from build123d import *

# Parameters (mm, degrees)
SKETCH1_R           = 1.75
SKETCH1_R_2         = 1.798521792
BOSS_EXTRUDE1_DEPTH = 5
SKETCH2_R           = 2.65
CUT_EXTRUDE1_DEPTH  = 3.5


with BuildPart() as part:
    # Sketch1 → Boss-Extrude1 (new body)
    with BuildSketch(Plane.YZ):
        Polygon((-67.5, -15.65), (-67.5, 15.65), (-60.8, 22.35), (-29.12737367, 22.35), (-21.9, 29.57737367), (-21.9, 35.8), (-15.2, 42.5), (15.2, 42.5), (21.9, 35.8), (21.9, 29.57737367), (29.12737367, 22.35), (60.8, 22.35), (67.5, 15.65), (67.5, -15.65), (60.8, -22.35), (29.12737367, -22.35), (21.9, -29.57737367), (21.9, -35.8), (15.2, -42.5), (-15.2, -42.5), (-21.9, -35.8), (-21.9, -29.57737367), (-29.12737367, -22.35), (-60.8, -22.35), align=None)
        with Locations(Location((0, 32.15, 0), (0, 0, 270))):
            Circle(SKETCH1_R, mode=Mode.SUBTRACT)
        with Locations(Location((-32.15, 0, 0), (0, 0, 270))):
            Circle(SKETCH1_R, mode=Mode.SUBTRACT)
        with Locations(Location((0, -32.15, 0), (0, 0, 270))):
            Circle(SKETCH1_R, mode=Mode.SUBTRACT)
        with Locations(Location((32.15, 0, 0), (0, 0, 270))):
            Circle(SKETCH1_R, mode=Mode.SUBTRACT)
        with Locations(Location((-62.5, -15, 0), (0, 0, 270))):
            Circle(SKETCH1_R, mode=Mode.SUBTRACT)
        with Locations(Location((-62.5, 15, 0), (0, 0, 270))):
            Circle(SKETCH1_R, mode=Mode.SUBTRACT)
        with Locations(Location((62.5, -15, 0), (0, 0, 90))):
            Circle(SKETCH1_R, mode=Mode.SUBTRACT)
        with Locations(Location((62.5, 15, 0), (0, 0, 90))):
            Circle(SKETCH1_R, mode=Mode.SUBTRACT)
        with Locations(Location((-15, 30, 0), (0, 0, 270))):
            Circle(SKETCH1_R_2, mode=Mode.SUBTRACT)
        with Locations(Location((15, 30, 0), (0, 0, 270))):
            Circle(SKETCH1_R_2, mode=Mode.SUBTRACT)
        with Locations(Location((15, -30, 0), (0, 0, 270))):
            Circle(SKETCH1_R_2, mode=Mode.SUBTRACT)
        with Locations(Location((-15, -30, 0), (0, 0, 270))):
            Circle(SKETCH1_R_2, mode=Mode.SUBTRACT)
        with BuildLine():
            Line((41, -16), (47.5, -16))
            ThreePointArc((47.5, -16), (49.621320344, -15.121320344), (50.5, -13))
            Line((50.5, -13), (50.5, 13))
            ThreePointArc((50.5, 13), (49.621320344, 15.121320344), (47.5, 16))
            Line((47.5, 16), (41, 16))
            ThreePointArc((41, 16), (38.878679656, 15.121320344), (38, 13))
            Line((38, 13), (38, -13))
            ThreePointArc((38, -13), (38.878679656, -15.121320344), (41, -16))
        make_face(mode=Mode.SUBTRACT)
        with BuildLine():
            Line((-41, -16), (-47.5, -16))
            ThreePointArc((-47.5, -16), (-49.621320344, -15.121320344), (-50.5, -13))
            Line((-50.5, -13), (-50.5, 13))
            ThreePointArc((-50.5, 13), (-49.621320344, 15.121320344), (-47.5, 16))
            Line((-47.5, 16), (-41, 16))
            ThreePointArc((-41, 16), (-38.878679656, 15.121320344), (-38, 13))
            Line((-38, 13), (-38, -13))
            ThreePointArc((-38, -13), (-38.878679656, -15.121320344), (-41, -16))
        make_face(mode=Mode.SUBTRACT)
    extrude(amount=BOSS_EXTRUDE1_DEPTH)

    # Sketch2 → Cut-Extrude1 (cut)
    with BuildSketch(Plane(origin=(0, 0, 0), x_dir=(0, -1, 0), z_dir=(-1, 0, 0))):
        with Locations(Location((-15, 30, 0), (0, 0, 90))):
            Circle(SKETCH2_R)
        with Locations(Location((15, 30, 0), (0, 0, 90))):
            Circle(SKETCH2_R)
        with Locations(Location((15, -30, 0), (0, 0, 90))):
            Circle(SKETCH2_R)
        with Locations(Location((-15, -30, 0), (0, 0, 90))):
            Circle(SKETCH2_R)
    extrude(amount=-CUT_EXTRUDE1_DEPTH, mode=Mode.SUBTRACT)


solid = part.part
Here's how the part is built. I have some questions about the finished solid (model axes, mm). A direction names the side the tool comes from. Give positions to 0.01 mm unless a question says otherwise; leave off trailing zeros. Order: outer loops, then holes, each group sorted by start corner. A loop starts at its lowest first (then second) coordinate and runs counter-clockwise, first axis right, second up. Notation, with made-up numbers: (-1, 20) -> (39, 20) arc R35 ccw to (39, 55) -> close; hole circle Ø8 at (15, 78.25). An arc over 180 degrees is marked (long way). One line per item, written item: value. Start each with the question number.
1. We'd pull the mould along Y, two halves only. Please class faces 4 (the face through (0, 1, 1)), 5 (the face through (2, -21.9, -33)), 6 (the face through (4.24, 16.517, -30.967)), 7 (the face through (2.46, 38.86, -15.1)): released by +Y, released by -Y, zero draft, split by the parting line, or undercut.
2. Imagine slicing it at C-C, the plane y = -62.5. List the corners of the cut face in (x, z) for me.
3. For faces 1 (the face through (1.726, 15.117, 27.353)), 2 (the face through (2.46, -49.64, 15.1)), 3 (the face through (2, 45, -22.35)), which set-ups out of +Z, -Z, +X, -X, +Y, -Y let a thin tool reach every point of the face, with its end or its side?
4. Will these pins go through, and if not, where does the flat tip stop? pin 1 Ø1.5 at (y, z) = (24, -32) entering from -X; pin 2 Ø2 at (x, y) = (2, 32.5) entering from -Z; pin 3 Ø2.5 at (x, y) = (3.5, 40.5) entering from +Z; pin 4 Ø3 at (x, z) = (3, 32) entering from -Y.
5. Imagine slicing it at B-B, the plane y = -32.15. List the corners of the cut face in (x, z) for me, plus the area to 3 significant figures.
6. I need wall thicknesses on probe 1 along Y at (x, z) = (4, 11); probe 2 along Z at (x, y) = (4.7, 15); probe 3 along Y at (x, z) = (1.2, 30). Which ranges of each line are inside material? Lowest first, please. Write a range as from..to.
7. Imagine slicing it at A-A, the plane z = 8. List the corners of the cut face in (x, y) for me.
8. Imagine slicing it at D-D, the plane x = 0.8. Count the separate pieces of the cut face and the enclosed holes in it, plus the area to 3 significant figures.
Values follow:
1. face 4: zero draft
1. face 5: released by -Y
1. face 6: undercut
1. face 7: undercut
2. outline: (0, -20.65) -> (5, -20.65) -> (5, -16.75) -> (0, -16.75) -> close; (0, -13.25) -> (5, -13.25) -> (5, 13.25) -> (0, 13.25) -> close; (0, 16.75) -> (5, 16.75) -> (5, 20.65) -> (0, 20.65) -> close
3. face 1: -X
3. face 2: +X, -X
3. face 3: -Z, +X, -X, +Y
4. pin 1: passes through
4. pin 2: stops at z = -22.35
4. pin 3: stops at z = 22.35
4. pin 4: stops at y = -21.9
5. outline: (0, -22.35) -> (5, -22.35) -> (5, -1.75) -> (0, -1.75) -> close; (0, 1.75) -> (5, 1.75) -> (5, 22.35) -> (0, 22.35) -> close
5. area: 206 mm2
6. probe 1: y = -67.5..-50.5, -38..38, 50.5..67.5
6. probe 2: z = -42.5..-31.8, -28.2..28.2, 31.8..42.5
6. probe 3: y = -21.9..-17.65, -12.35..12.35, 17.65..21.9
7. outline: (0, -67.5) -> (5, -67.5) -> (5, -50.5) -> (0, -50.5) -> close; (0, -38) -> (5, -38) -> (5, 38) -> (0, 38) -> close; (0, 50.5) -> (5, 50.5) -> (5, 67.5) -> (0, 67.5) -> close
8. separate pieces: 1
8. enclosed holes: 14
8. area: 6,770 mm2
